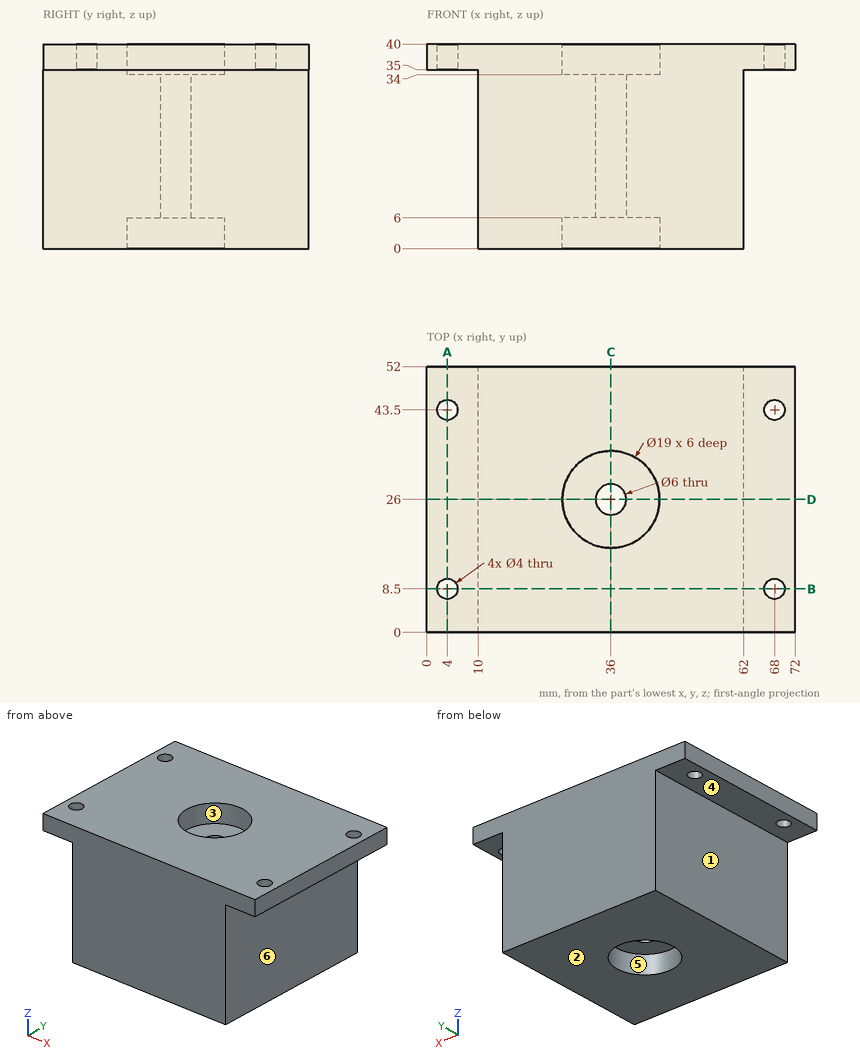
The figure shows three views and two pictorial views of one solid part (mm, origin at its lowest corner). Answer the questions. A direction names the side the tool comes from. Give positions to 0.01 mm unless a question says otherwise; leave off trailing zeros. Write each loop counter-clockwise with the first axis right and the second up, starting at its lowest first coordinate (ties: lowest second). Pieces come first, ordered by that corner, then holes. Notation, with made-up numbers: M -1,66.5 L 20,66.5 A12 ccw 20,81.5 Z; hole C 16,63 d6. An arc over 180 degrees is marked long. One line per item, written item: value. Start each with the question number.
(1) Find the intervals of material crossed by line 1 (Y direction, x = 68, z = 37); line 2 (Y direction, x = 36, z = 2.4); line 3 (X direction, y = 43, z = 38), in increasing order.
(2) Find section C-C (x = 36). Determine the outline of the cut face in (y, z).
(3) Determine the mould class of the marked faces 4, 5 and 6 for opening direction X: pulls with the +X half, pulls with the -X half, needs draft (parallel to the pull), parting line crosses it, or undercut.
(4) A tool of negligible diameter and unlimited length cuts with its end or side. For the marked faces 1, 2 and 3, from which of +Z, -Z, +X, -X, +Y, -Y can it reach the whole face along a straight path? Write none if from no direction.
(5) Find section B-B (y = 8.5). Determine the outline of the cut face in (x, z).
(6) Find section D-D (y = 26). Determine the outline of the cut face in (x, z).
(7) Flat-ended cylindrical pins translate along their axes: pin 1 Ø5 at (x, y) = (4, 43.5) entering from +Z; pin 2 Ø10 at (y, z) = (26.5, 22) entering from +X; pin 3 Ø4.5 at (x, y) = (68, 43.5) entering from -Z; pin 4 Ø15 at (x, y) = (36, 26) entering from +Z. Find the tip coordinate at first contact, or state that the pin passes through.
(8) Find section A-A (x = 4). Determine the outline of the cut face in (y, z).
Results below:
1. line 1: y = 0 to 6.5, 10.5 to 41.5, 45.5 to 52
1. line 2: y = 0 to 16.5, 35.5 to 52
1. line 3: x = 0 to 2.06, 5.94 to 66.06, 69.94 to 72
2. outline: M 0,0 L 16.5,0 L 16.5,6 L 23,6 L 23,34 L 16.5,34 L 16.5,40 L 0,40 Z; M 29,6 L 35.5,6 L 35.5,0 L 52,0 L 52,40 L 35.5,40 L 35.5,34 L 29,34 Z
3. face 4: needs draft
3. face 5: undercut
3. face 6: pulls with the +X half
4. face 1: -Z, -X, +Y, -Y
4. face 2: -Z, +X, -X, +Y, -Y
4. face 3: +Z
5. outline: M 0,35 L 2,35 L 2,40 L 0,40 Z; M 6,35 L 10,35 L 10,0 L 62,0 L 62,35 L 66,35 L 66,40 L 6,40 Z; M 70,35 L 72,35 L 72,40 L 70,40 Z
6. outline: M 0,35 L 10,35 L 10,0 L 26.5,0 L 26.5,6 L 33,6 L 33,34 L 26.5,34 L 26.5,40 L 0,40 Z; M 39,6 L 45.5,6 L 45.5,0 L 62,0 L 62,35 L 72,35 L 72,40 L 45.5,40 L 45.5,34 L 39,34 Z
7. pin 1: stops at z = 40
7. pin 2: stops at x = 62
7. pin 3: stops at z = 35
7. pin 4: stops at z = 34
8. outline: M 0,35 L 6.5,35 L 6.5,40 L 0,40 Z; M 10.5,35 L 41.5,35 L 41.5,40 L 10.5,40 Z; M 45.5,35 L 52,35 L 52,40 L 45.5,40 Z
